Verification items for the finished model (mm, model axes). A direction names the side the tool comes from. Give positions to 0.01 mm unless a question says otherwise; leave off trailing zeros. Order: outer loops, then holes, each group sorted by start corner. A loop starts at its lowest first (then second) coordinate and runs counter-clockwise, first axis right, second up. Notation, with made-up numbers: (31.5, 18) -> (40.5, 18) arc R24 ccw to (40.5, 31) -> close; hole circle Ø8 at (79.5, 50.25). An arc over 180 degrees is marked (long way). Return JSON: item names as keys, results as strings. Group by question number.
(1) Depth check by flat-ended pin: pin 1 Ø5 at (x, z) = (-2, 39) entering from +Y; pin 2 Ø4 at (x, y) = (-4.5, -12.5) entering from -Z; pin 3 Ø1.6 at (x, y) = (1, 17) entering from +Z; pin 4 Ø7.5 at (x, y) = (-5, 6.5) entering from -Z. Enter the tip coordinate at first touch or a pass-through.
(2) Cross-section at B-B on y = -14. Enter the section's corners in (x, z), then the cut area to 3 significant figures.
(3) Cross-section at C-C on x = -7.5. Enter the section's corners in (y, z), then the cut area to 3 significant figures.
(4) Cross-section at A-A on z = 89.5. Enter the section's corners in (x, y), then the cut area to 3 significant figures.
(5) Thickness scan on line 1 along Y through (x, z) = (-10.5, 179.5); line 2 along Z through (x, y) = (-2.25, 14); line 3 along Z through (x, y) = (-0.25, 10). Record the ranges inside material, lowest first.
(6) Tool access check on faces 1 (the face through (-6, -1.984, 174)), 2 (the face through (-0.6, -13.14, 219.61)), 3 (the face through (-0.43, 14.094, 195.254)), 4 (the face through (1.984, 8, 174)), 5 (the face through (-0.43, -1.937, 80.679)). Record the directions out of +Z, -Z, +X, -X, +Y, -Y that give a thin tool (end or side, any length) a straight path to the whole face; none if there is none.
from build123d import *

# Parameters (mm, degrees)
SKETCH1_R                = 1.984375
BOSS_EXTRUDE1_DEPTH      = 170
BOSS_EXTRUDE2_DEPTH      = 15
BOSS_EXTRUDE2_DEPTH_BACK = 6.35
SKETCH2_W                = 15
SKETCH2_H                = 20
SKETCH3_R                = 1.984375
BOSS_EXTRUDE3_DEPTH      = 20.799999976
SKETCH4_R                = 1.984375
REVOLVE5_ANGLE           = 90
SKETCH6_R                = 1.984375
BOSS_EXTRUDE4_DEPTH      = 35.000000038


with BuildPart() as part:
    # Sketch1 → Boss-Extrude1 (new body)
    with BuildSketch(Plane.XY):
        Circle(SKETCH1_R)
    extrude(amount=BOSS_EXTRUDE1_DEPTH)

    # Sketch2 → Boss-Extrude2 (add, two sides: drawn at the far end of the back side and taken through both)
    with BuildSketch(Plane.XY.offset(170).offset(-BOSS_EXTRUDE2_DEPTH_BACK)):
        with Locations((-5.515625, 8.015625)):
            Rectangle(SKETCH2_W, SKETCH2_H)
    extrude(amount=BOSS_EXTRUDE2_DEPTH + BOSS_EXTRUDE2_DEPTH_BACK)

    # Sketch3 → Boss-Extrude3 (add)
    with BuildSketch(Plane.XY.offset(185)):
        with Locations((0, 16.03125)):
            Circle(SKETCH3_R)
    extrude(amount=BOSS_EXTRUDE3_DEPTH)

    # Sketch4 → Revolve5 (revolve)
    with BuildSketch(Plane.XY.offset(205.799999976)):
        with Locations(Location((0, 16.03125, 0), (0, 0, 90))):
            Circle(SKETCH4_R)
    revolve(axis=Axis((-5.972283048, 4.112992181, 205.799999976), (1, 0, 0)), revolution_arc=REVOLVE5_ANGLE)

    # Sketch6 → Boss-Extrude4 (add)
    with BuildSketch(Plane.XZ.offset(-4.112992181)):
        with Locations(Location((0, 217.718257795, 0), (0, 0, 90))):
            Circle(SKETCH6_R)
    extrude(amount=BOSS_EXTRUDE4_DEPTH)


solid = part.part
Verdict:
{
 "1": {"pin 1": "y = 1.98", "pin 2": "through", "pin 3": "z = 212.3", "pin 4": "z = 163.65"},
 "2": {"outline": "circle Ø3.97 at (0, 217.72)", "area": "12.4 mm²"},
 "3": {"outline": "(-1.98, 163.65) -> (18.02, 163.65) -> (18.02, 185) -> (-1.98, 185) -> close", "area": "427 mm²"},
 "4": {"outline": "circle Ø3.97 at (0, 0)", "area": "12.4 mm²"},
 "5": {"line 1": "-1.98 to 18.02", "line 2": "163.65 to 185", "line 3": "163.65 to 185, 213.82 to 218.38"},
 "6": {"face 1": "-Z, +X, -X, -Y", "face 2": "-Y", "face 3": "none", "face 4": "+Z, -Z, +X, +Y, -Y", "face 5": "-Z"}
}
